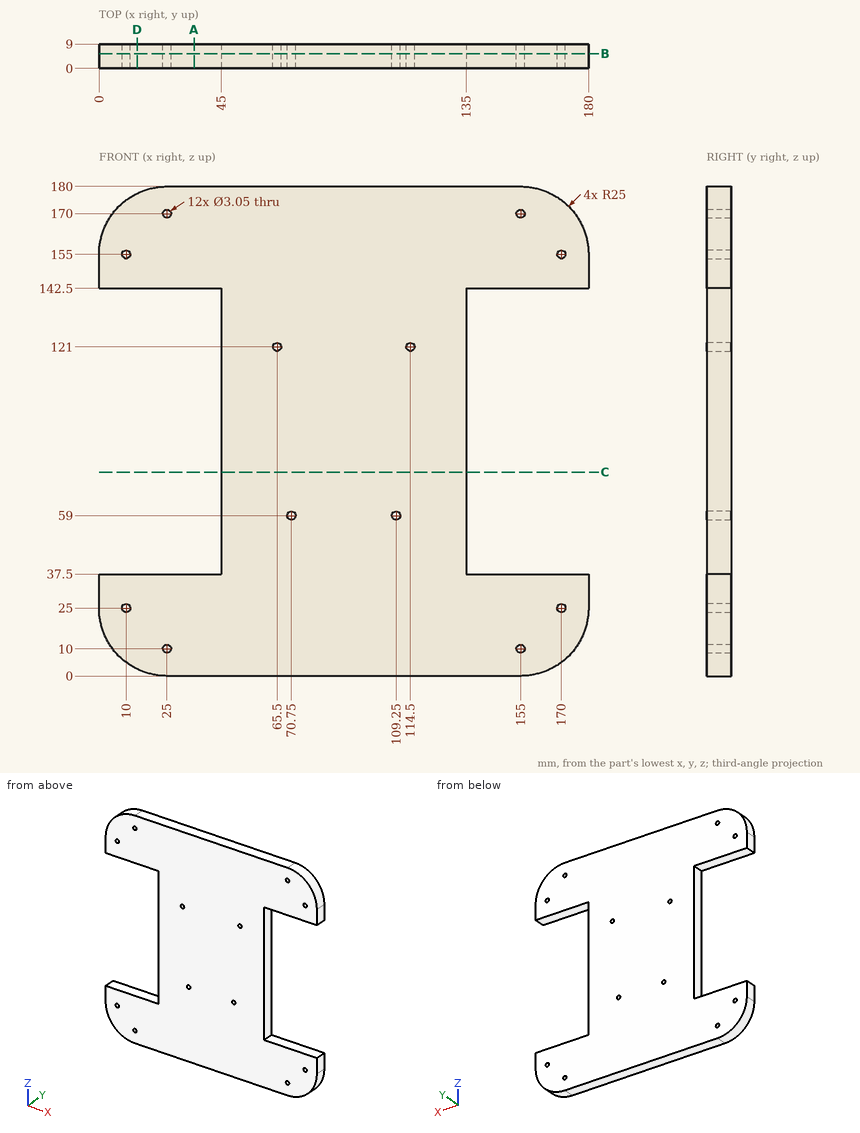
Check sheet for the drawn part. Datum: minimum x, y, z corner. Units: mm. Coordinates: 2 decimals unless noted, no trailing zeros. Order: outer loops, then holes, each group sorted by start corner. A loop starts at its lowest first (then second) coordinate and runs counter-clockwise, first axis right, second up. Notation, with made-up numbers: M 9.5,-25.5 L 16.5,-25.5 A28 cw 16.5,-2.5 Z; hole C 49.5,-30.5 d2. An arc over 180 degrees is marked long. One line per question, with ' | ' between items. Start each with the question number.
Item 1: Gauge pin test, flat ends, axial feed: pin 1 (5 mm diameter, centred on x = 25, z = 170, fed in from +Y); pin 2 (1.5 mm diameter, centred on y = 3.5, z = 76.5, fed in from -X); pin 3 (4.5 mm diameter, centred on y = 4.5, z = 77.5, fed in from +X); pin 4 (4.5 mm diameter, centred on x = 22, y = 4, fed in from +Z). Record the tip position at first contact, or that the pin passes through.
Item 2: Cross-section at D-D on x = 14. Enter the section's corners in (y, z), then the cut area to 3 significant figures.
Item 3: Cross-section at A-A on x = 35. Enter the section's corners in (y, z).
Item 4: Cross-section at C-C on z = 75. Enter the section's corners in (x, y), then the cut area to 3 significant figures.
Item 5: Cross-section at B-B on y = 5.5. State how many separate pieces and enclosed holes the cut face has, then the cut area to 3 significant figures.
Item 6: Material ranges on L1, parallel to Z at x = 155, y = 4.75 (3 decimals); L2, parallel to X at y = 5.25, z = 155 (3 decimals); L3, parallel to X at y = 3, z = 170 (3 decimals), recorded low to high. Write a range as [from, to].
Findings:
1) pin 1: stops at y = 9 | pin 2: stops at x = 45 | pin 3: stops at x = 135 | pin 4: stops at z = 179.99
2) outline: M 0,2.55 L 9,2.55 L 9,37.5 L 0,37.5 Z; M 0,142.5 L 9,142.5 L 9,177.45 L 0,177.45 Z | area: 629 mm²
3) outline: M 0,0 L 9,0 L 9,37.5 L 0,37.5 Z; M 0,142.5 L 9,142.5 L 9,180 L 0,180 Z
4) outline: M 45,0 L 135,0 L 135,9 L 45,9 Z | area: 810 mm²
5) separate pieces: 1 | enclosed holes: 12 | area: 22,300 mm²
6) L1: z = [0, 8.475], [11.525, 37.5], [142.5, 168.475], [171.525, 180] | L2: x = [0, 8.475], [11.525, 168.475], [171.525, 180] | L3: x = [5, 23.475], [26.525, 153.475], [156.525, 175]
